Can you work these out from the drawing? Everything is in mm from the part's minimum corner. Give positions to 0.01 mm unless a question says otherwise; leave off trailing zeros. Order: outer loops, then holes, each group sorted by start corner. A loop starts at its lowest first (then second) coordinate and runs counter-clockwise, first axis right, second up. Notation, with made-up numbers: (-19.75, 3) -> (15.25, 3) arc R25 ccw to (15.25, 37) -> close; hole circle Ø11 at (9.25, 36.25). An arc over 180 degrees is marked (long way). Answer as CSV lines item,"result". Start each with the question number.
(1) I want a section at D-D (z = 5). Give the number of separate pieces and of enclosed holes in the cut face, plus the area to 4 significant figures.
(2) I need wall thicknesses on L1, parallel to Y at x = 25, z = 17.9; L2, parallel to X at y = 15, z = 9. Which ranges of each line are inside material? Lowest first, please.
(3) We'd pull the mould along X, two halves only. Please class the marked faces 1, 2, 3 and 4: released by +X, released by -X, zero draft, split by the parting line, or undercut.
(4) I want a section at A-A (y = 1). Please give me the cut outline in (x, z).
(5) I want a section at C-C (x = 11.25). Please give me the cut outline in (y, z).
(6) Will these pins go through, and if not, where does the flat tip stop? pin 1 Ø4 at (y, z) = (15, 15) entering from +X; pin 2 Ø3 at (x, y) = (15, 5) entering from -Z.
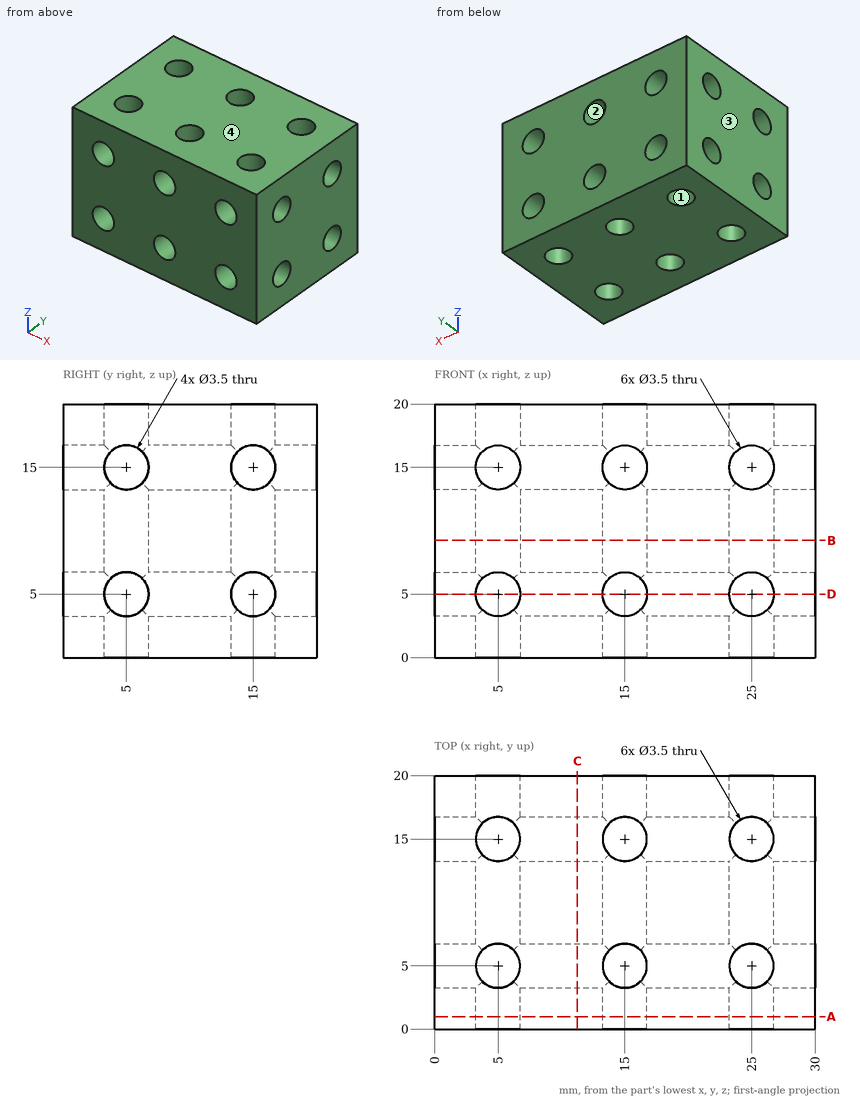
Final values:
1,separate pieces,"12"
1,enclosed holes,"0"
1,area,"253.5 mm²"
2,L1,"0 to 3.25, 6.75 to 13.25, 16.75 to 20"
2,L2,"0 to 3.25, 6.75 to 13.25, 16.75 to 23.25, 26.75 to 30"
3,face 1,"undercut"
3,face 2,"undercut"
3,face 3,"released by -X"
3,face 4,"zero draft"
4,outline,"(0, 0) -> (30, 0) -> (30, 20) -> (0, 20) -> close; hole circle Ø3.5 at (5, 5); hole circle Ø3.5 at (5, 15); hole circle Ø3.5 at (15, 5); hole circle Ø3.5 at (15, 15); hole circle Ø3.5 at (25, 5); hole circle Ø3.5 at (25, 15)"
5,outline,"(0, 0) -> (20, 0) -> (20, 20) -> (0, 20) -> close; hole circle Ø3.5 at (5, 5); hole circle Ø3.5 at (5, 15); hole circle Ø3.5 at (15, 5); hole circle Ø3.5 at (15, 15)"
6,pin 1,"x = 30"
6,pin 2,"through"
